Source: CAD feature listing. Evaluate the final solid. Frame: model axes, mm. A direction names the side the tool comes from. Coordinates: 2 decimals unless noted, no trailing zeros. Loops run counter-clockwise (first coordinate to the right, second up) from the corner with the lowest first, then second, coordinate; pieces in that order, holes last. Notation, with made-up numbers: M 70,58.25 L 106,58.25 A18 ccw 106,76.25 Z; hole C 9,14.25 d11. An arc over 180 degrees is marked long. One line per question, with ' | ' between items. Start each with the question number.
1. Pin query (flat end, axial travel): P1, Ø8, axis at x = 16.98, z = 64.3, coming from the +Y side. Return the tip coordinate at first contact, or that it passes through.
2. Ray query, probe 1 along Y at (x, z) = (23, 67.5); probe 2 along Z at (x, y) = (26, 2.75); probe 3 along X at (y, z) = (2, 26). Return the intervals inside material, ascending.
3. Access query for faces 1 (the flat face through (24.977, 0.362, 56.738)), 2 (the flat face through (33, 6, 59)). Directions: +Z, -Z, +X, -X, +Y, -Y. A direction counts if a zero-diameter tool reaches every point of the face in a straight line with its end or side. Return the directions, or none.
4. Mould query, pull axis X, two halves, no side actions, for faces 3 (the cylindrical face through (35.556, 4.479, 60.447)), 4 (the cylindrical face through (17.73, 1.48, 66.68)), 5 (the flat face through (25, 0, 61)), 6 (the cylindrical face through (28.189, 1.479, 66.795)). Classes: pulls with the +X half, pulls with the -X half, needs draft (parallel to the pull), parting line crosses it, or undercut.
5. Section query A-A, the plane y = 4.25. Output: boundary loops of the cut face in (x, z).
```python
from build123d import *

# Parameters (mm, degrees)
EXTRUDE_2_DEPTH          = 3
SKETCH_6_R               = 2.5
CUT_EXTRUDE_3_DEPTH      = 3
FILLET_1_R               = 5
EXTRUDE_START            = 3
SKETCH_12_R              = 2.5
EXTRUDE_3_DEPTH          = 3
CUT_EXTRUDE_4_DEPTH      = 53.075400229
CUT_EXTRUDE_4_DEPTH_BACK = 53.075400229


with BuildPart() as part:
    # 草图5 → 凸台-拉伸2 (new body)
    with BuildSketch(Plane(origin=(0, 0, 0), x_dir=(1, 0, 0), z_dir=(0, 1, 0))):
        with BuildLine():
            ThreePointArc((10.559870576, -71.726836912), (50.703091685, -51.821293824), (71.479455105, -12.121777836))
            add(Edge.make_bspline(
                [(0, 0), (21.999765175, 5.26655471), (58.910704789, -3.551422078), (71.479455105, -12.121777836)],
                knots=[0, 0, 0, 0, 1, 1, 1, 1], degree=3))
            add(Edge.make_bspline(
                [(0, 0), (11.807092486, -19.295565119), (14.826805821, -57.124859445), (10.559870576, -71.726836912)],
                knots=[0, 0, 0, 0, 1, 1, 1, 1], degree=3))
        make_face()
    extrude(amount=EXTRUDE_2_DEPTH)

    # 草图6 → 切除-拉伸3 (cut)
    with BuildSketch(Plane(origin=(0, 0, 0), x_dir=(1, 0, 0), z_dir=(0, 1, 0))):
        with Locations(Location((16.980367579, -64.295545078, 0), (0, 0, 270))):
            Circle(SKETCH_6_R)
        with BuildLine():
            Line((10.193167245, 1.43451668), (79.733938156, 38.033041096))
            Line((79.733938156, 38.033041096), (67.619590309, -86.298423653))
            Line((67.619590309, -86.298423653), (37.943421347, -61.778206323))
            add(Edge.make_bspline(
                [(10.193167245, 1.43451668), (25.470457842, -12.985420951), (40.3134982, -34.977892419), (37.943421347, -61.778206323)],
                knots=[0, 0, 0, 0, 1, 1, 1, 1], degree=3))
        make_face()
    extrude(amount=CUT_EXTRUDE_3_DEPTH, mode=Mode.SUBTRACT)

    # 圆角1
    fillet_1_edges = [part.edges().sort_by_distance(p)[0] for p in [
        (10.559870576, 1.5, 71.726836912),
    ]]
    fillet(fillet_1_edges, radius=FILLET_1_R)

    # 草图12 → 凸台-拉伸3 (add)
    with BuildSketch(Plane(origin=(0, 0, 0), x_dir=(1, 0, 0), z_dir=(0, 1, 0)).offset(EXTRUDE_START)):
        with Locations(Location((33.447510377, -59.102789962, 0), (0, 0, 270))):
            Circle(SKETCH_12_R)
    extrude(amount=EXTRUDE_3_DEPTH)

    # 草图15 → 切除-拉伸4 (cut, two sides: drawn at the far end of the back side and taken through both)
    with BuildSketch(Plane(origin=(20.307849495, 0, 46.141092032), x_dir=(-0.3007418808113313, 0, -0.9537055736054305), z_dir=(0.9537055736054305, 0, -0.3007418808113313)).offset(-CUT_EXTRUDE_4_DEPTH_BACK)):
        Polygon((-11.510635463, 0.734616999), (50.112437496, 2.140825412), (51.673202283, 2.140825412), (51.673202283, -11.401301697), (-11.510635463, -3.981764366), align=None)
    extrude(amount=CUT_EXTRUDE_4_DEPTH + CUT_EXTRUDE_4_DEPTH_BACK, mode=Mode.SUBTRACT)


solid = part.part
```
Taken from the geometry:
1) P1: y = 3
2) probe 1: 0 to 3 | probe 2: 17.35 to 67.68 | probe 3: 9.38 to 30.92
3) face 1: -Z, -X, -Y | face 2: +Z, -Z, +X, -X, +Y
4) face 3: parting line crosses it | face 4: undercut | face 5: needs draft | face 6: pulls with the +X half
5) outline: C 33.45,59.1 d5
